CAD build for the part. Positions are in the model's coordinates, mm. Give positions to 0.01 mm unless a question says otherwise; leave off trailing zeros. Loops run counter-clockwise (first coordinate to the right, second up) from the corner with the lowest first, then second, coordinate; pieces in that order, holes last. Notation, with made-up numbers: M -39,21 L 13,21 A32 ccw 13,58 Z; hole C -8.75,-25 d2. An arc over 180 degrees is marked long. Answer as CSV lines item,"result".
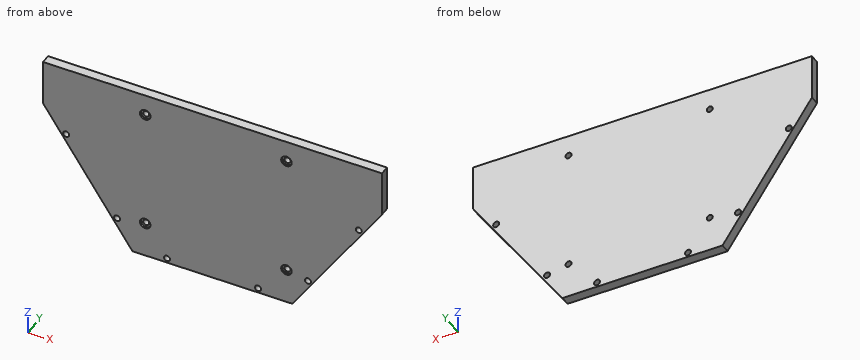
from build123d import *

# Parameters (mm, degrees)
BOSS_EXTRUDE1_DEPTH = 5
SKETCH2_R           = 1.6
CUT_EXTRUDE1_DEPTH  = 10
SKETCH3_R           = 1.6
CUT_EXTRUDE2_DEPTH  = 13
SKETCH5_R           = 2.8
CUT_EXTRUDE3_DEPTH  = 1
SKETCH4_R           = 2.8
CUT_EXTRUDE4_DEPTH  = 1


with BuildPart() as part:
    # Sketch1 → Boss-Extrude1 (new body)
    with BuildSketch(Plane(origin=(0, 0, 0), x_dir=(1, 0, 0), z_dir=(0, 1, 0))):
        Polygon((44.733199147, 23.708961101), (-40.266800853, 23.708961101), (-87.761294074, -46.784110287), (-87.761294074, -71.294110287), (92.227692368, -71.294110287), (92.227692368, -46.784110287), align=None)
    extrude(amount=BOSS_EXTRUDE1_DEPTH)

    # Sketch2 → Cut-Extrude1 (cut)
    with BuildSketch(Plane(origin=(0, 5, 0), x_dir=(1, 0, 0), z_dir=(0, 1, 0))):
        with Locations((-21.927484651, 21.208961101)):
            Circle(SKETCH2_R)
        with Locations((26.393882946, 21.208961101)):
            Circle(SKETCH2_R)
        with Locations((-48.443257362, 7.098961101)):
            Circle(SKETCH2_R)
        with Locations((-75.438186307, -32.967904005)):
            Circle(SKETCH2_R)
        with Locations((52.909655656, 7.098961101)):
            Circle(SKETCH2_R)
        with Locations((79.904584601, -32.967904005)):
            Circle(SKETCH2_R)
    extrude(amount=-CUT_EXTRUDE1_DEPTH, mode=Mode.SUBTRACT)

    # Sketch3 → Cut-Extrude2 (cut)
    with BuildSketch(Plane(origin=(0, 5, 0), x_dir=(1, 0, 0), z_dir=(0, 1, 0))):
        with Locations((-33.49256942, 4.708961101)):
            Circle(SKETCH3_R)
        with Locations((41.50743058, 4.708961101)):
            Circle(SKETCH3_R)
        with Locations((41.50743058, -59.791038899)):
            Circle(SKETCH3_R)
        with Locations((-33.49256942, -59.791038899)):
            Circle(SKETCH3_R)
    extrude(amount=-CUT_EXTRUDE2_DEPTH, mode=Mode.SUBTRACT)

    # Sketch5 → Cut-Extrude3 (cut)
    with BuildSketch(Plane(origin=(0, 0, 0), x_dir=(-1, 0, 0), z_dir=(0, -1, 0))):
        with Locations((33.49256942, 4.708961101)):
            Circle(SKETCH5_R)
        with Locations((33.49256942, -59.791038899)):
            Circle(SKETCH5_R)
        with Locations((-41.50743058, -59.791038899)):
            Circle(SKETCH5_R)
    extrude(amount=-CUT_EXTRUDE3_DEPTH, mode=Mode.SUBTRACT)

    # Sketch4 → Cut-Extrude4 (cut)
    with BuildSketch(Plane.XZ):
        with Locations((41.50743058, -4.708961101)):
            Circle(SKETCH4_R)
    extrude(amount=-CUT_EXTRUDE4_DEPTH, mode=Mode.SUBTRACT)


solid = part.part
1) Band-saw the part on C-C on z = -10.5. Give the cut face in (x, y), and give its area (3 significant figures).
Answer below:
outline,"M -49.17,0 L 53.63,0 L 53.63,5 L -49.17,5 Z"
area,"514 mm^2"
2) Drill centre lines: line 1 (X direction, y = 1.35, z = -3.5); line 2 (X direction, y = 3.8, z = -8.5); line 3 (Z direction, x = 26, y = 4.7). Where is each one in solid material? Low to high. Write a range as from..to.
Answer below:
line 1,"x = -53.88..-34.54, -32.44..40.46, 42.56..58.35"
line 2,"x = -50.51..-49.22, -47.67..52.14, 53.68..54.98"
line 3,"z = -23.71..-22.76, -19.66..71.29"
3) Band-saw the part on A-A on y = 2.05. Give the number of separate pieces and of enclosed holes in the cut face, and give its area (3 significant figures).
Answer below:
separate pieces,"1"
enclosed holes,"10"
area,"13,700 mm^2"
4) Band-saw the part on B-B on z = 23. Give the cut face in (x, y).
Answer below:
outline,"M -71.74,0 L 76.2,0 L 76.2,5 L -71.74,5 Z"
5) Flat gauge pins, fed straight in: pin 1 (4.5 mm diameter, centred on x = 41.51, z = -4.71, fed in from -Y); pin 2 (1.5 mm diameter, centred on y = 3.5, z = 4.5, fed in from +X); pin 3 (1.5 mm diameter, centred on y = 3, z = 37, fed in from +X); pin 4 (1.9 mm diameter, centred on x = -21.93, z = -21.21, fed in from +Y). Where does each tip first touch, or does it go through?
Answer below:
pin 1,"stops at y = 1"
pin 2,"stops at x = 64.24"
pin 3,"stops at x = 86.14"
pin 4,"passes through"
